Check sheet for the modelled part. Datum: model origin and axes. Units: mm. Round coordinates to 2 decimals unless told otherwise and drop trailing zeros. Write each loop counter-clockwise with the first axis right and the second up, starting at its lowest first coordinate (ties: lowest second). Pieces come first, ordered by that corner, then holes. Notation, with made-up numbers: M 86.25,-15 L 91.25,-15 A25 ccw 91.25,21 Z; hole C 78,36.5 d6. An arc over 180 degrees is marked long. Put each result on its own line as item: value.
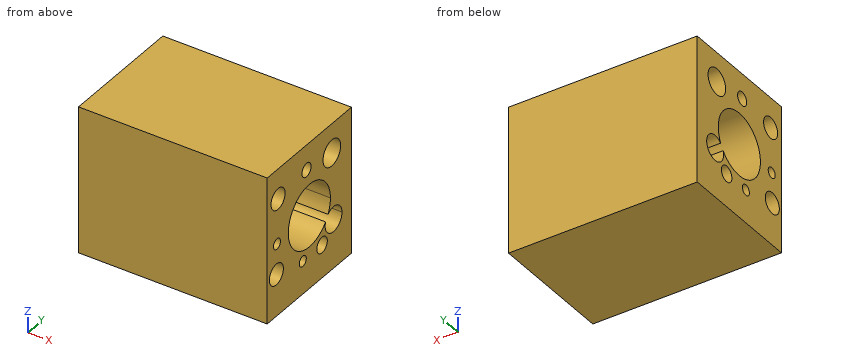
```python
from build123d import *

# Parameters (mm, degrees)
F0_W     = 114.3
F0_H     = 88.9
F1_DEPTH = 76.2
F2_R     = 6.35
F2_R_2   = 7.9375
F2_R_3   = 3.175
F2_R_4   = 4.1275
F2_R_5   = 4.7625
F3_DEPTH = 114.3


with BuildPart() as f1:
    # F0 (on Front) → F1 (new body)
    with BuildSketch(Plane.XZ):
        with Locations((3.3618031452, -5.2332123742)):
            Rectangle(F0_W, F0_H)
    extrude(amount=F1_DEPTH)

    # F2 (on face) → F3 (cut, through all)
    with BuildSketch(Plane.YZ.offset(60.5118031452)):
        with BuildLine():
            ThreePointArc((-21.2015970146, -14.027896936), (-19.5957156735, -9.7602380604), (-19.05, -5.2332123742))
            ThreePointArc((-19.05, -5.2332123742), (-56.0237840544, 1.2197299913), (-23.4217023803, -17.3761147861))
            ThreePointArc((-23.4217023803, -17.3761147861), (-22.5362767831, -15.5530622079), (-21.2015970146, -14.027896936))
        make_face()
        with BuildLine():
            ThreePointArc((-21.2015970146, -14.027896936), (-22.5362767831, -15.5530622079), (-23.4217023803, -17.3761147861))
            ThreePointArc((-23.4217023803, -17.3761147861), (-22.2231411807, -15.7606932709), (-21.2015970146, -14.027896936))
        make_face()
        with BuildLine():
            ThreePointArc((-21.2015970146, -14.027896936), (-22.2231411807, -15.7606932709), (-23.4217023803, -17.3761147861))
            ThreePointArc((-23.4217023803, -17.3761147861), (-17.3948287668, -27.2874849256), (-8.5655332553, -19.7640545666))
            ThreePointArc((-8.5655332553, -19.7640545666), (-13.0357718235, -12.82550984), (-21.2015970146, -14.027896936))
        make_face()
        with Locations((-66.3864538074, 20.9288746119)):
            Circle(F2_R)
        with Locations((-17.78, 21.4367876258)):
            Circle(F2_R_2)
        with Locations((-67.9182708263, -24.1526439786)):
            Circle(F2_R)
        with Locations((-67.3732608557, -5.9233275242)):
            Circle(F2_R_3)
        with Locations((-44.0157242119, -29.6750832349)):
            Circle(F2_R_3)
        with Locations((-40.64, 23.9767876258)):
            Circle(F2_R_4)
        with Locations((-26.6011171043, -29.6750832349)):
            Circle(F2_R_5)
    extrude(amount=-F3_DEPTH, mode=Mode.SUBTRACT)


solid = f1.part
```
1. Cross-section at C-C (x = -30). Count the separate pieces of the cut face and the enclosed holes in it, then the cut area to 3 significant figures.
Computed values:
separate pieces: 1
enclosed holes: 8
area: 4,810 mm2
2. Cross-section at B-B (z = 11.5). Enter the section's corners in (x, y).
Computed values:
outline: M -53.79,-76.2 L 60.51,-76.2 L 60.51,-47.21 L -53.79,-47.21 Z; M -53.79,-28.99 L 60.51,-28.99 L 60.51,0 L -53.79,0 Z
3. Scan lines: probe 1 along Y at (x, z) = (-39, -25.5); probe 2 along Z at (x, y) = (-1.5, -46); probe 3 along Z at (x, y) = (45, -66.5). Record each from-to range of solid material in increasing order.
Computed values:
probe 1: y = -76.2 to -74.12, -61.71 to -28.89, -24.31 to -21.2, -11.17 to 0
probe 2: z = -49.68 to -32.15, -27.2 to -22.57, 12.1 to 39.22
probe 3: z = -49.68 to -30.34, -17.96 to -8.98, -2.87 to 14.58, 27.28 to 39.22
4. Cross-section at A-A (y = -38.1). Enter the section's corners in (x, z), then the cut area to 3 significant figures.
Computed values:
outline: M -53.79,-49.68 L 60.51,-49.68 L 60.51,-24.28 L -53.79,-24.28 Z; M -53.79,13.82 L 60.51,13.82 L 60.51,20.72 L -53.79,20.72 Z; M -53.79,27.23 L 60.51,27.23 L 60.51,39.22 L -53.79,39.22 Z
area: 5,060 mm2
5. Depth check by flat-ended pin: pin 1 Ø24.5 at (y, z) = (-16.19, -19.76) entering from -X. Enter the tip coordinate at first touch or a pass-through.
Computed values:
pin 1: stops at x = -53.79
